Geometry: see drawing. Coordinates: mm, zero at the bounding-box minimum. A direction names the side the tool comes from. Round coordinates to 2 decimals unless told otherwise and drop trailing zeros. Loops run counter-clockwise (first coordinate to the right, second up) from the corner with the lowest first, then second, coordinate; pieces in that order, holes last. Notation, with made-up numbers: (15, 40.5) - (69, 40.5) arc R18 ccw to (69, 66.5) - close; hole circle Ø2 at (65.25, -33). An arc over 180 degrees is marked (long way). Return JSON: item names as keys, results as strings. Group by question number.
1. Section D-D on y = 5.75. Return loops of the section in (x, z), and give its area (3 significant figures).
2. Set-up query: the marked faces 1, 2 and 3. Return all of +Z, -Z, +X, -X, +Y, -Y with unobstructed straight access to the full face (end or side cutting, diameter ignored); none if empty.
3. Section B-B on x = 3.5. Return loops of the section in (y, z), and give its area (3 significant figures).
4. Section A-A on z = 71. Return loops of the section in (x, y).
5. Section C-C on x = 22.5. Return loops of the section in (y, z), and give its area (3 significant figures).
6. First-contact query: pin 1 Ø2.5 at (x, z) = (22.5, 48) entering from +Y; pin 2 Ø6 at (x, z) = (69.5, 69.5) entering from +Y; pin 3 Ø4 at (x, z) = (22.5, 32) entering from +Y; pin 4 Ø4.5 at (y, z) = (10.5, 72.5) entering from +X. Flat tips, straight axial feed; report the tip coordinate or a pass-through.
7. Material intervals for probe 1 along Z at (x, y) = (119.5, 0.55); probe 2 along X at (y, z) = (0.6, 48); probe 3 along X at (y, z) = (6.75, 69), sorted ascending.
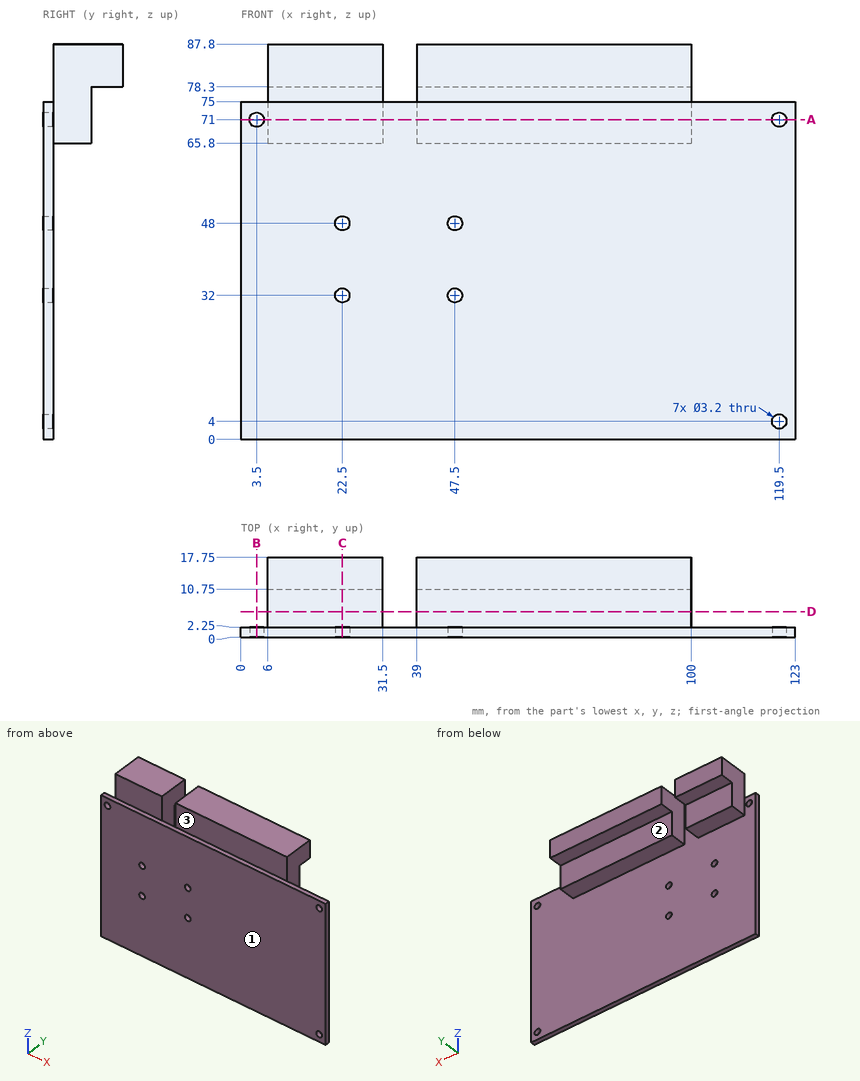
Taken from the geometry:
{
 "1": {"outline": "(6, 65.8) - (31.5, 65.8) - (31.5, 87.8) - (6, 87.8) - close; (39, 65.8) - (100, 65.8) - (100, 87.8) - (39, 87.8) - close", "area": "1,900 mm2"},
 "2": {"face 1": "+Z, -Z, +X, -X, -Y", "face 2": "-Z, +X, -X, +Y", "face 3": "+Z, +X, -X, -Y"},
 "3": {"outline": "(0, 0) - (2.25, 0) - (2.25, 69.4) - (0, 69.4) - close; (0, 72.6) - (2.25, 72.6) - (2.25, 75) - (0, 75) - close", "area": "162 mm2"},
 "4": {"outline": "(0, 0) - (1.9, 0) - (1.9, 2.25) - (0, 2.25) - close; (5.1, 0) - (117.9, 0) - (117.9, 2.25) - (100, 2.25) - (100, 10.75) - (39, 10.75) - (39, 2.25) - (31.5, 2.25) - (31.5, 10.75) - (6, 10.75) - (6, 2.25) - (5.1, 2.25) - close; (121.1, 0) - (123, 0) - (123, 2.25) - (121.1, 2.25) - close"},
 "5": {"outline": "(0, 0) - (2.25, 0) - (2.25, 30.4) - (0, 30.4) - close; (0, 33.6) - (2.25, 33.6) - (2.25, 46.4) - (0, 46.4) - close; (0, 49.6) - (2.25, 49.6) - (2.25, 65.8) - (10.75, 65.8) - (10.75, 78.3) - (17.75, 78.3) - (17.75, 87.8) - (2.25, 87.8) - (2.25, 75) - (0, 75) - close", "area": "408 mm2"},
 "6": {"pin 1": "through", "pin 2": "y = 10.75", "pin 3": "y = 2.25", "pin 4": "x = 100"},
 "7": {"probe 1": "0 to 2.4, 5.6 to 69.4, 72.6 to 75", "probe 2": "0 to 20.9, 24.1 to 45.9, 49.1 to 123", "probe 3": "6 to 31.5, 39 to 100"}
}
